Design review of the part built by this model. Coordinates are the model's own, in mm. A direction names the side the tool comes from. Give positions to 0.01 mm unless a question says otherwise; leave off trailing zeros. Loops run counter-clockwise (first coordinate to the right, second up) from the corner with the lowest first, then second, coordinate; pieces in that order, holes last. Notation, with made-up numbers: (40.5, 79) -> (64.5, 79) arc R12 ccw to (64.5, 102) -> close; hole circle Ø8 at (-10.5, 9.5). An arc over 180 degrees is marked (long way). Use a Markdown table: item, result. Add a question column.
1. For faces 4 (the flat face through (-6.676, 5.991, -49.71)), 5 (the flat face through (20, 6, 56.9)), 6 (the flat face through (1, 9.895, 37)), list the 3-axis set-ups (+Z, -Z, +X, -X, +Y, -Y) from which the entire face can be reached by the end or side of a thin tool; tool diameter is ignored.
2. Add section C-C (z = -32.5). State the section outline as (x, y) points (3 decimals), and give its area (3 significant figures).
3. Add section A-A (x = 20). State the section outline as (y, z) points.
4. Draft analysis for pull direction Y (two halves, no side actions). For faces 1 (the flat face through (-17.4, 7, 62)), 2 (the flat face through (-20, 0, -2)), 3 (the flat face through (2.875, 8, 37)), state which applies: pulls with the +Y half, pulls with the -Y half, needs draft (parallel to the pull), parting line crosses it, or undercut.
5. For pin 1 Ø1.5 at (x, y) = (19, 7) entering from +Z; pin 2 Ø1.7 at (x, y) = (-19, 3.5) entering from +Z; pin 3 Ø5 at (x, y) = (-2.5, 8.5) entering from -Z; pin 4 Ø1 at (x, z) = (1, 37.5) entering from -Y (3 decimals), all flat-tipped, find the tip position at first contact; note any pin that passes through.
6. To check wall thickness, follow line 1 (X direction, y = 5, z = 3); line 2 (Z direction, x = -5, y = 8); line 3 (X direction, y = 4, z = 37.5). State the ranges of each line that lie inside material, in increasing order.
Autodesk Inventor part; units mm, degrees
ref_plane "Work Plane1" through (20, 0, 0) normal (1, 0, 0) x (0, 1, 0)
ref_plane "XZ Plane" through (0, 0, 0) normal (0, 1, 0) x (-1, 0, 0)
ref_plane "XY Plane" through (0, 0, 0) normal (0, 0, 1) x (1, 0, 0)
sketch "Sketch1" plane through (0, 0, 0) normal (0, 0, 1) x (1, 0, 0)
  line L0 (0, 0) -> (0, 44.0101) construction
  line L1 (-33.5, 0) -> (-6.975, 0)
  line L2 (6.975, 0) -> (33.5, 0)
  arc A0 (6.975, 0) -> (-6.975, 0) centre (0, 0) ccw
  line L3 (33.5, 0) -> (33.5, 20.5)
  line L4 (33.5, 20.5) -> (-33.5, 20.5)
  line L5 (-33.5, 20.5) -> (-33.5, 0)
ref_plane "Work Plane1" through (20, 0, 0) normal (1, 0, 0) x (0, 1, 0)
extrude "Extrusion3" add sketch "Sketch1" along normal mid plane 129
sketch "Sketch4" plane through (20, 0, 0) normal (1, 0, 0) x (0, 1, 0)
  line L0 (0, 64.5) -> (0, -64.5)
  line L1 (2, 64.6) -> (10.1, 64.6)
  arc A0 (8, 56.9) -> (9.8375, 57.9834) centre (8, 59) ccw
  line L2 (8, 56.9) -> (4.9024, 56.9)
  arc A1 (6.2736, 58.9704) -> (4.9024, 56.9) centre (7, 57) ccw
  line L3 (6.9278, 59.9087) -> (6.9278, 60.4)
  line L4 (5.4278, 61.9) -> (2, 61.9)
  arc A2 (2, 61.9) -> (0.1051, 60.1387) centre (2, 60) ccw
  line L5 (0.1051, 60.1387) -> (0, 58.7036)
  line L6 (0, 62.6) -> (0, 58.7036)
  line L7 (0, -64.5) -> (0, 64.5)
  arc A3 (2, 64.6) -> (0, 62.6) centre (2, 62.6) ccw
  arc A4 (6.9278, 60.4) -> (5.4278, 61.9) centre (5.4278, 60.4) ccw
  line L8 (9.8375, 57.9834) -> (13.4982, 64.6)
  line L9 (13.4982, 64.6) -> (10.1, 64.6)
  arc A5 (6.2736, 58.9704) -> (6.9278, 59.9087) centre (5.9278, 59.9087) ccw
  point P0 (0, 0)
  point P1 (0, 64.6)
  point P2 (8, 64.6)
  point P3 (10.1, 62.5)
  point P4 (6.9278, 59.0988)
  point P5 (6.9278, 61.9)
  point P6 (0, 62.6)
  dimension "d33" = 2
  dimension "d34" = 1.5
  dimension "d35" = 1
extrude "Extrusion4" cut sketch "Sketch4" along normal mid plane 5.2
mirror "Mirror2" about plane through (0, 0, 0) normal (1, 0, 0) of "Extrusion4"
sketch "Sketch5" plane through (33.5, 0, 64.5) normal (1, 0, 0) x (0, 0, -1)
  line L0 (1.9, 0) -> (5.7964, 0)
  arc A0 (0, 2.5) -> (2.5, 0) centre (2.5, 2.5) ccw
  line L1 (2.5, 2.5) -> (2.5, 0) construction
  line L2 (2.5, 2.5) -> (5, 2.5) construction
  line L3 (2.5, 2.5) -> (0, 2.5) construction
  line L4 (0, 0) -> (0, 20.5)
  line L5 (0, 2.5) -> (0, 0)
  line L6 (0, 0) -> (129, 0)
  point P0 (64.5, 0)
  dimension "d36" = 90
  dimension "d37" = 90
  dimension "d38" = 2.5
extrude "Extrusion5" cut sketch "Sketch5" against normal through all
sketch "Sketch6" plane through (0, 0, 64.5) normal (0, 0, 1) x (1, 0, 0)
  arc A0 (6.5116, 2.5) -> (-6.5116, 2.5) centre (0, 0) ccw
  line L0 (0, 6.975) -> (2.875, 6.975) construction
  line L1 (2.875, 6.975) -> (2.875, 9.895) construction
  line L2 (-17.4, 0) -> (-6.975, 0)
  line L3 (2.875, 9.895) -> (2.875, 6.3549)
  spline S0 degree 6 poles (-6.5116, 2.5) (-6.5776, 2.3279) (-6.6388, 2.1522) (-6.6938, 1.976) (-6.7418, 1.8023) (-6.7828, 1.6341) (-6.8262, 1.4334) (-6.8346, 1.3932) (-6.8426, 1.3535) (-6.8502, 1.3144) (-6.8574, 1.2759) (-6.8768, 1.1683) (-6.8881, 1.1008) (-6.8982, 1.0356) (-6.9073, 0.9727) (-6.9153, 0.9122) (-6.9314, 0.7817) (-6.939, 0.7131) (-6.9453, 0.6483) (-6.9506, 0.5874) (-6.955, 0.5303) (-6.9696, 0.3178) (-6.9738, 0.1923) (-6.9749, 0.099) (-6.975, 0.0363) (-6.975, 0.0034) (-6.975, 0.0002) knots 0 0 0 0 0 0 0 0.246271 0.246271 0.246271 0.246271 0.246271 0.309061 0.309061 0.309061 0.309061 0.309061 0.424616 0.424616 0.424616 0.424616 0.424616 0.569008 0.569008 0.569008 0.569008 0.569008 1 1 1 1 1 1 1
  line L4 (2.875, 9.895) -> (-0.5799, 9.895)
  line L5 (-2.875, 9.895) -> (-2.875, 8.895) construction
  arc A1 (-2.409, 9.2729) -> (-5.2406, 6.1296) centre (4.7239, 0) ccw
  arc A2 (-0.5799, 9.895) -> (-2.409, 9.2729) centre (-0.5799, 6.895) ccw
  line L6 (-6.5813, 2.3101) -> (-5.2406, 6.1296)
  point P0 (-1.5174, 9.895)
  dimension "d41" = 2.875
  dimension "d42" = 2.92
  dimension "d50" = 5.75
  dimension "d52" = 3
sketch "Sketch7" plane through (0, 0, -64.5) normal (0, 0, -1) x (-1, 0, 0)
  arc A0 (6.975, 0) -> (-6.975, 0) centre (0, 0) ccw construction
  line L0 (0, 6.975) -> (-2.25, 6.975) construction
  line L1 (-2.25, 6.975) -> (-2.25, 10.675) construction
  arc A1 (8.1198, 7.2861) -> (-2.25, 10.675) centre (0, 0) ccw
  line L2 (0, 0) -> (8.1198, 7.2861) construction
  line L3 (0, 0) -> (-2.25, 10.675) construction
  line L4 (-2.25, 10.675) -> (-2.25, 6.6021)
  line L5 (8.1198, 7.2861) -> (5.1914, 4.6583)
  arc A2 (5.1914, 4.6583) -> (-2.25, 6.6021) centre (0, 0) ccw
  dimension "d45" = 2.25
  dimension "d46" = 3.7
  dimension "d47" = 60
extrude "Extrusion7" cut sketch "Sketch7" against normal blind 30
extrude "Extrusion8" cut sketch "Sketch6" against normal blind 56.46
properties part number "Laser_Pen_Housing_Top"
Taken from the geometry:
| question | item | result |
|---|---|---|
| 1 | face 4 | -Z |
| 1 | face 5 | none |
| 1 | face 6 | +Z, -Y |
| 2 | outline | (-33.5, 0) -> (-6.975, 0) arc R6.975 cw to (6.975, 0) -> (33.5, 0) -> (33.5, 20.5) -> (-33.5, 20.5) -> close |
| 2 | area | 1,300 mm^2 |
| 3 | outline | (0, -64.5) -> (20.5, -64.5) -> (20.5, 64.5) -> (13.44, 64.5) -> (9.84, 57.98) arc R2.1 cw to (8, 56.9) -> (4.9, 56.9) arc R2.1 cw to (6.27, 58.97) arc R1 ccw to (6.93, 59.91) -> (6.93, 60.4) arc R1.5 ccw to (5.43, 61.9) -> (2, 61.9) arc R1.9 ccw to (0.11, 60.14) -> (0, 58.7) -> close |
| 4 | face 1 | undercut |
| 4 | face 2 | pulls with the -Y half |
| 4 | face 3 | needs draft |
| 5 | pin 1 | stops at z = 61.65 |
| 5 | pin 2 | stops at z = 61.9 |
| 5 | pin 3 | stops at z = -64.5 |
| 5 | pin 4 | stops at y = 9.895 |
| 6 | line 1 | x = -33.5 to -4.86, 4.86 to 33.5 |
| 6 | line 2 | z = -34.5 to 64.5 |
| 6 | line 3 | x = -33.5 to -5.99, 5.71 to 33.5 |
